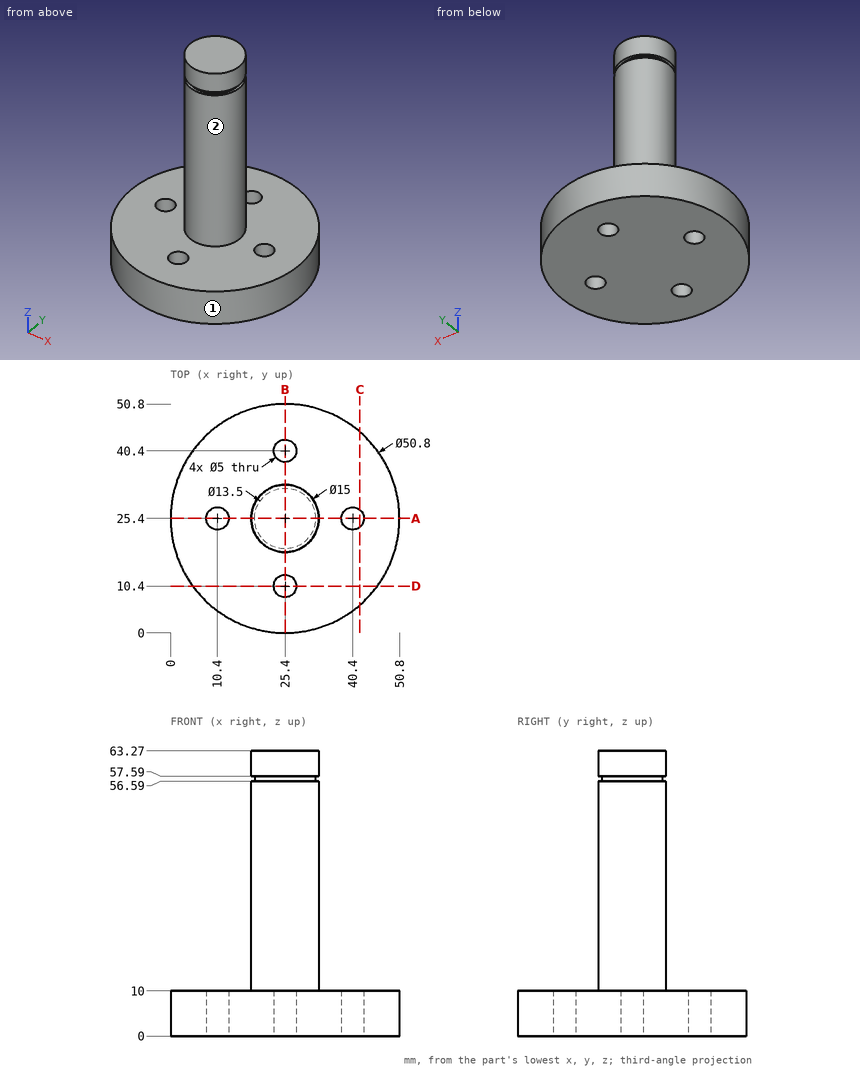
Study the drawing (mm; zero at the part's minimum x, y, z) and answer. A direction names the side the tool comes from. Give positions to 0.01 mm unless a question says otherwise; leave off trailing zeros. Write each loop counter-clockwise with the first axis right and the second up, starting at its lowest first coordinate (ties: lowest second). Pieces come first, ordered by that corner, then holes.
Item 1: Section A-A, the plane y = 25.4 is taken. Write down the section's boundary in (x, z), plus the area to 3 significant figures.
Item 2: Which of the six approach directions +Z, -Z, +X, -X, +Y, -Y give full straight-line access (tool end or side, diameter ignored) to the marked faces 1 and 2?
Item 3: Section D-D, the plane y = 10.4 is taken. Write down the section's boundary in (x, z).
Item 4: Flat-ended cylindrical pins translate along their axes: P1, Ø10, axis at x = 15, z = 32, coming from the +Y side; P2, Ø10, axis at y = 20, z = 22, coming from the +X side; P3, Ø4, axis at y = 42.5, z = 7.5, coming from the +X side. Find the tip coordinate at first contact, or state that the pin passes through.
Item 5: Find the intervals of material crossed by line 1 along Y through (x, z) = (25.4, 5.25); line 2 along Z through (x, y) = (30, 12.5); line 3 along Y through (x, z) = (10.4, 3.75), in increasing order.
Item 6: Section C-C, the plane x = 42 is taken. Write down the section's boundary in (y, z), plus the area to 3 significant figures.
Completed:
1. outline: (0, 0) - (7.9, 0) - (7.9, 10) - (0, 10) - close; (12.9, 0) - (37.9, 0) - (37.9, 10) - (32.9, 10) - (32.9, 56.59) - (32.15, 56.59) - (32.15, 57.59) - (32.9, 57.59) - (32.9, 63.27) - (17.9, 63.27) - (17.9, 57.59) - (18.65, 57.59) - (18.65, 56.59) - (17.9, 56.59) - (17.9, 10) - (12.9, 10) - close; (42.9, 0) - (50.8, 0) - (50.8, 10) - (42.9, 10) - close
1. area: 1,210 mm2
2. face 1: +Z, -Z
2. face 2: +Z
3. outline: (4.9, 0) - (22.9, 0) - (22.9, 10) - (4.9, 10) - close; (27.9, 0) - (45.9, 0) - (45.9, 10) - (27.9, 10) - close
4. P1: stops at y = 30.6
4. P2: stops at x = 32.89
4. P3: stops at x = 45.82
5. line 1: y = 0 to 7.9, 12.9 to 37.9, 42.9 to 50.8
5. line 2: z = 0 to 10
5. line 3: y = 4.9 to 22.9, 27.9 to 45.9
6. outline: (6.18, 0) - (23.48, 0) - (23.48, 10) - (6.18, 10) - close; (27.32, 0) - (44.62, 0) - (44.62, 10) - (27.32, 10) - close
6. area: 346 mm2
